Could you check a few things on this model? Use its own coordinates, in mm. Face numbers are marked on the shaded views. A direction names the side the tool comes from. Give positions to 0.01 mm unless a question says otherwise; leave off trailing zeros. Order: outer loops, then holes, each group sorted by start corner. A loop starts at its lowest first (then second) coordinate and runs counter-clockwise, first axis right, second up.
(1) Imagine slicing it at C-C, the plane x = 0. Write out the boundary of the cut face in (y, z) (3 decimals), then the cut area to 3 significant figures.
(2) If I drill on probe 1 along Y at (x, z) = (0, 8.25) (3 decimals); probe 2 along Y at (x, z) = (-13, 4.5) (3 decimals); probe 3 along Y at (x, z) = (-17, 5.75), over which ranges is the centre line in solid material (lowest first)?
(3) If we mould it in two halves opening along Y, with no side actions, what happens to the marked faces 5, 6 and 7? For each: released by +Y, released by -Y, zero draft, split by the parting line, or undercut.
(4) On a 3-axis mill with a long thin cutter (end or side, diameter ignored), from which of +Z, -Z, +X, -X, +Y, -Y can I reach the whole of each face in a straight line? I mean the marked faces 1, 2, 3 and 4. Say none if no direction works.
(5) Imagine slicing it at A-A, the plane y = 1. Write out the boundary of the cut face in (x, z).
(6) Imagine slicing it at D-D, the plane z = 10.25. Write out the boundary of the cut face in (x, y) (3 decimals), then the cut area to 3 significant figures.
(7) Imagine slicing it at B-B, the plane x = -15.5. Write out the boundary of the cut face in (y, z), then the cut area to 3 significant figures.
(8) Will these pins go through, and if not, where does the flat tip stop? pin 1 (3 mm diameter, centred on x = 25.5, z = 2, fed in from +Y); pin 2 (1.5 mm diameter, centred on x = 3.5, z = 7.5, fed in from +Y); pin 3 (3 mm diameter, centred on x = 24, z = 3.5, fed in from -Y).
from build123d import *

# Parameters (mm, degrees)
BOSS_EXTRUDE1_DEPTH         = 6.35
CIRPATTERN1_COUNT           = 5
SKETCH3_R                   = 6.35
BOSS_EXTRUDE2_DEPTH         = 4.826
F_1_4_0_25_DIAMETER_HOLE1_D = 6.35


with BuildPart() as part:
    # Sketch2 → Boss-Extrude1 (new body)
    with BuildSketch(Plane.XY):
        with BuildLine():
            Line((4.12074162, 12.682338645), (0, 0))
            Line((0, 0), (13.335, 0))
            ThreePointArc((13.335, 0), (14.078948776, 1.796051224), (15.875, 2.54))
            Line((15.875, 2.54), (31.265996882, 2.54))
            ThreePointArc((31.265996882, 2.54), (31.014248813, 4.704309891), (30.612864998, 6.845922701))
            ThreePointArc((30.612864998, 6.845922701), (18.47357946, 13.421841122), (15.970754926, 26.999058282))
            ThreePointArc((15.970754926, 26.999058282), (14.057994528, 28.042591729), (12.077407934, 28.950826907))
            Line((12.077407934, 28.950826907), (7.321328337, 14.31311903))
            ThreePointArc((7.321328337, 14.31311903), (6.058780655, 12.834865625), (4.12074162, 12.682338645))
        make_face()
    boss_extrude1 = extrude(amount=BOSS_EXTRUDE1_DEPTH)

    # CirPattern1: Boss-Extrude1 ×5 about axis
    cirpattern1_axis = Axis((0, 0, 0), (0, 0, 1))
    for i in range(1, CIRPATTERN1_COUNT):
        add(boss_extrude1.rotate(cirpattern1_axis, i * 360 / CIRPATTERN1_COUNT))

    # Sketch3 → Boss-Extrude2 (add)
    with BuildSketch(Plane.XY.offset(6.35)):
        Circle(SKETCH3_R)
    extrude(amount=BOSS_EXTRUDE2_DEPTH)

    # 1/4 (0.25) Diameter Hole1 (through all)
    with Locations(Plane.XY.offset(11.176)):
        with Locations((0, 0)):
            Hole(F_1_4_0_25_DIAMETER_HOLE1_D / 2)


solid = part.part
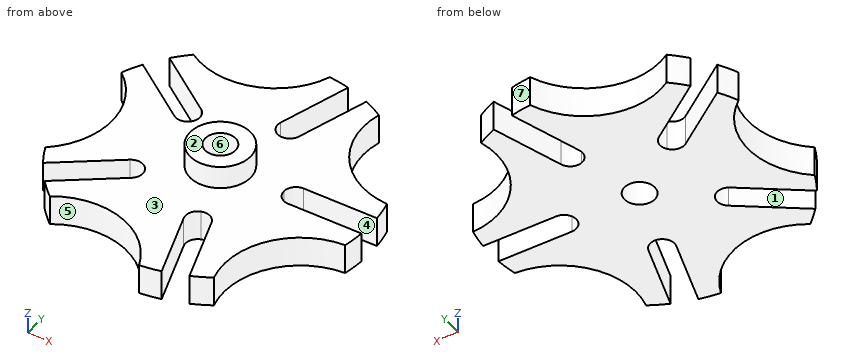
Answer block:
1. outline: (-26.351, 0) - (-3.175, 0) - (-3.175, 11.176) - (-6.35, 11.176) - (-6.35, 6.35) - (-26.351, 6.35) - close; (3.175, 0) - (26.351, 0) - (26.351, 6.35) - (6.35, 6.35) - (6.35, 11.176) - (3.175, 11.176) - close
1. area: 325 mm2
2. probe 1: y = -6.35 to -3.175, 3.175 to 6.35
2. probe 2: y = -20.965 to -12.585, -6.796 to 6.796, 12.585 to 20.965
2. probe 3: y = -21.73 to -15.49, -9.21 to 9.21, 15.49 to 21.73
3. face 5: released by -Y
3. face 6: undercut
3. face 7: released by +Y
4. face 1: +Z, -Z
4. face 2: +Z, +X, -X, +Y, -Y
4. face 3: +Z
4. face 4: +Z, -Z, +X
5. outline: (-22.87, 0) - (-3.01, 0) - (-3.01, 11.18) - (-6.27, 11.18) - (-6.27, 6.35) - (-22.87, 6.35) - close; (3.01, 0) - (13.54, 0) - (13.54, 6.35) - (6.27, 6.35) - (6.27, 11.18) - (3.01, 11.18) - close
6. outline: circle Ø12.7 at (0, 0); hole circle Ø6.35 at (0, 0)
6. area: 95.0 mm2
7. outline: (-21.32, 0) - (-14.4, 0) - (-14.4, 6.35) - (-21.32, 6.35) - close; (-8.12, 0) - (8.12, 0) - (8.12, 6.35) - (-8.12, 6.35) - close; (14.4, 0) - (21.32, 0) - (21.32, 6.35) - (14.4, 6.35) - close
7. area: 191 mm2
8. pin 1: stops at y = 8.65
8. pin 2: stops at y = 5.72
8. pin 3: stops at y = -9.54
